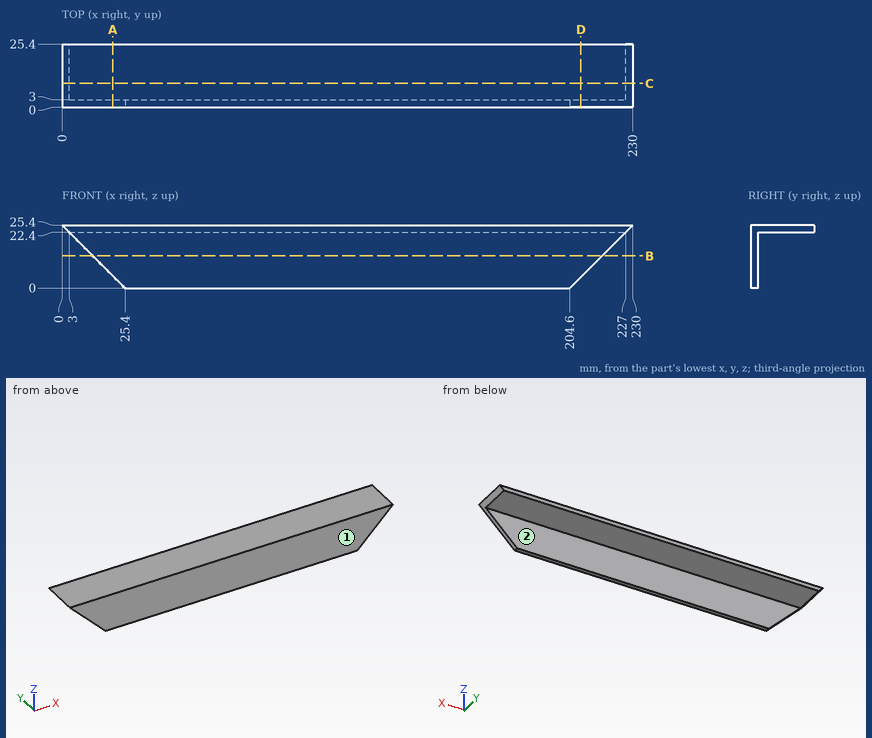
Part print with two shaded views. Sizes in mm from the minimum x, y, z corner. A direction names the side the tool comes from. Coordinates: 2 decimals unless noted, no trailing zeros. Write each loop counter-clockwise with the first axis right and the second up, starting at its lowest first coordinate (ties: lowest second). Pieces come first, ordered by that corner, then holes.
(1) 3-axis set-ups, long thin cutter, end or side, ignore diameter. For the marked faces 1 and 2: which of +Z, -Z, +X, -X, +Y, -Y reach the whole face in a straight line?
(2) Cut at D-D on x = 209. List the corners of the cut face in (y, z).
(3) Pin check, flat tips, straight feed: pin 1 Ø1 at (x, z) = (173, 19.5) entering from +Y; pin 2 Ø12 at (x, y) = (122, 13) entering from -Z. Stop position of each tip, or through.
(4) Drill centre lines: line 1 (Z direction, x = 135.5, y = 13.75); line 2 (Y direction, x = 198, z = 20); line 3 (X direction, y = 2, z = 5.75). Where is each one in solid material? Low to high.
(5) Cut at A-A on x = 20.5. List the corners of the cut face in (y, z), and give its area (3 significant figures).
(6) Cut at C-C on y = 9.5. List the corners of the cut face in (x, z).
(7) Cut at B-B on z = 13. List the corners of the cut face in (x, y), and give its area (3 significant figures).
Working result:
1. face 1: +Z, -Z, +X, -X, -Y
1. face 2: -Z, +X, -X, +Y
2. outline: (0, 4.4) - (3, 4.4) - (3, 22.4) - (25.4, 22.4) - (25.4, 25.4) - (0, 25.4) - close
3. pin 1: stops at y = 3
3. pin 2: stops at z = 22.4
4. line 1: z = 22.4 to 25.4
4. line 2: y = 0 to 3
4. line 3: x = 19.65 to 210.35
5. outline: (0, 4.9) - (3, 4.9) - (3, 22.4) - (25.4, 22.4) - (25.4, 25.4) - (0, 25.4) - close
5. area: 129 mm2
6. outline: (0, 25.4) - (3, 22.4) - (227, 22.4) - (230, 25.4) - close
7. outline: (12.4, 0) - (217.6, 0) - (217.6, 3) - (12.4, 3) - close
7. area: 616 mm2
